The model under review builds one solid part; all positions refer to its coordinate system, in mm. Coordinates: 2 decimals unless noted, no trailing zeros. Order: outer loops, then holes, each group sorted by start corner. A loop starts at its lowest first (then second) coordinate and runs counter-clockwise, first axis right, second up. Notation, with made-up numbers: M 54.5,3 L 74.5,3 A25 cw 74.5,20 Z; hole C 41,10 d7. An arc over 180 degrees is marked long. Answer as CSV lines item,"result". Start each with the question number.
Q1. For P1, Ø10, axis at x = 14.5, y = 2, coming from the +Z side; P2, Ø2, axis at y = 2, z = 1.5, coming from the -X side (3 decimals); P3, Ø3, axis at y = 9.5, z = 2, coming from the +X side; P4, Ø1, axis at y = 9.5, z = 1.5, coming from the +X side, all flat-tipped, find the tip position at first contact; note any pin that passes through.
Q2. Wall thickness on L1, parallel to X at y = 15.5, z = 2.25; L2, parallel to Y at x = 7.5, z = 2.25; L3, parallel to Y at x = -11.5, z = 4.9: over which ranges is each line inside the solid? List them lowest first. Write a range as [from, to].
Q3. Consider section B-B on y = 5. Write out the cut boundary in (x, z), and give its area (3 significant figures).
Q4. Consider section A-A on x = 0. Write out the cut boundary in (y, z).
Q5. Consider section C-C on y = -8.5. Write out the cut boundary in (x, z), and give its area (3 significant figures).
Q6. Consider section D-D on x = -8. Write out the cut boundary in (y, z).
from build123d import *

# Parameters (mm, degrees)
SKETCH1_R           = 20
BOSS_EXTRUDE1_DEPTH = 6


with BuildPart() as part:
    # Sketch1 → Boss-Extrude1 (new body)
    with BuildSketch(Plane.XY):
        Circle(SKETCH1_R)
        with BuildLine():
            Line((-2, -2.236067977), (2, -2.236067977))
            ThreePointArc((2, -2.236067977), (0, 3), (-2, -2.236067977))
        make_face(mode=Mode.SUBTRACT)
        with BuildLine():
            Line((-16.568425726, -3.806214518), (-5.988664565, -0.368641735))
            ThreePointArc((-5.988664565, -0.368641735), (-6, 0), (-5.988664565, 0.368641735))
            Line((-5.988664565, 0.368641735), (-16.568425726, 3.806214518))
            ThreePointArc((-16.568425726, 3.806214518), (-17, 0), (-16.568425726, -3.806214518))
        make_face(mode=Mode.SUBTRACT)
        with BuildLine():
            Line((-1.5, -16.933694222), (-1.5, -5.809475019))
            ThreePointArc((-1.5, -5.809475019), (-1.854101966, -5.706339098), (-2.201198248, -5.581641897))
            Line((-2.201198248, -5.581641897), (-8.739850239, -14.581324281))
            ThreePointArc((-8.739850239, -14.581324281), (-5.253288904, -16.167960777), (-1.5, -16.933694222))
        make_face(mode=Mode.SUBTRACT)
        with BuildLine():
            Line((1.5, -16.933694222), (1.5, -5.809475019))
            ThreePointArc((1.5, -5.809475019), (1.854101966, -5.706339098), (2.201198248, -5.581641897))
            Line((2.201198248, -5.581641897), (8.739850239, -14.581324281))
            ThreePointArc((8.739850239, -14.581324281), (5.253288904, -16.167960777), (1.5, -16.933694222))
        make_face(mode=Mode.SUBTRACT)
        with BuildLine():
            Line((-1.5, 5.809475019), (-1.5, 16.933694222))
            ThreePointArc((-1.5, 16.933694222), (-5.253288904, 16.167960777), (-8.739850239, 14.581324281))
            Line((-8.739850239, 14.581324281), (-2.201198248, 5.581641897))
            ThreePointArc((-2.201198248, 5.581641897), (-1.854101966, 5.706339098), (-1.5, 5.809475019))
        make_face(mode=Mode.SUBTRACT)
        with BuildLine():
            Line((-5.061613582, 3.221811284), (-15.641374743, 6.659384067))
            ThreePointArc((-15.641374743, 6.659384067), (-13.753288904, 9.992349289), (-11.166901222, 12.817968525))
            Line((-11.166901222, 12.817968525), (-4.628249231, 3.818286141))
            ThreePointArc((-4.628249231, 3.818286141), (-4.854101966, 3.526711514), (-5.061613582, 3.221811284))
        make_face(mode=Mode.SUBTRACT)
        with BuildLine():
            Line((-15.641374743, -6.659384067), (-5.061613582, -3.221811284))
            ThreePointArc((-5.061613582, -3.221811284), (-4.854101966, -3.526711514), (-4.628249231, -3.818286141))
            Line((-4.628249231, -3.818286141), (-11.166901222, -12.817968525))
            ThreePointArc((-11.166901222, -12.817968525), (-13.753288904, -9.992349289), (-15.641374743, -6.659384067))
        make_face(mode=Mode.SUBTRACT)
        with BuildLine():
            Line((11.166901222, 12.817968525), (4.628249231, 3.818286141))
            ThreePointArc((4.628249231, 3.818286141), (4.854101966, 3.526711514), (5.061613582, 3.221811284))
            Line((5.061613582, 3.221811284), (15.641374743, 6.659384067))
            ThreePointArc((15.641374743, 6.659384067), (13.753288904, 9.992349289), (11.166901222, 12.817968525))
        make_face(mode=Mode.SUBTRACT)
        with BuildLine():
            Line((8.739850239, 14.581324281), (2.201198248, 5.581641897))
            ThreePointArc((2.201198248, 5.581641897), (1.854101966, 5.706339098), (1.5, 5.809475019))
            Line((1.5, 5.809475019), (1.5, 16.933694222))
            ThreePointArc((1.5, 16.933694222), (5.253288904, 16.167960777), (8.739850239, 14.581324281))
        make_face(mode=Mode.SUBTRACT)
        with BuildLine():
            Line((15.641374743, -6.659384067), (5.061613582, -3.221811284))
            ThreePointArc((5.061613582, -3.221811284), (4.854101966, -3.526711514), (4.628249231, -3.818286141))
            Line((4.628249231, -3.818286141), (11.166901222, -12.817968525))
            ThreePointArc((11.166901222, -12.817968525), (13.753288904, -9.992349289), (15.641374743, -6.659384067))
        make_face(mode=Mode.SUBTRACT)
        with BuildLine():
            Line((16.568425726, -3.806214518), (5.988664565, -0.368641735))
            ThreePointArc((5.988664565, -0.368641735), (6, 0), (5.988664565, 0.368641735))
            Line((5.988664565, 0.368641735), (16.568425726, 3.806214518))
            ThreePointArc((16.568425726, 3.806214518), (17, 0), (16.568425726, -3.806214518))
        make_face(mode=Mode.SUBTRACT)
    extrude(amount=BOSS_EXTRUDE1_DEPTH)


solid = part.part
Evaluation:
1,P1,"stops at z = 6"
1,P2,"stops at x = -19.975"
1,P3,"stops at x = 18.33"
1,P4,"stops at x = 17.86"
2,L1,"x = [-12.64, -6.98], [-1.5, 1.5], [6.98, 12.64]"
2,L2,"y = [-18.54, -15.26], [-12.87, -7.77], [-4.01, -0.86], [0.86, 4.01], [7.77, 12.87], [15.26, 18.54]"
2,L3,"y = [-16.36, -12.52], [-5.31, -2.16], [2.16, 5.31], [12.52, 16.36]"
3,outline,"M -19.36,0 L -10.53,0 L -10.53,6 L -19.36,6 Z; M -5.49,0 L 5.49,0 L 5.49,6 L -5.49,6 Z; M 10.53,0 L 19.36,0 L 19.36,6 L 10.53,6 Z"
3,area,"172 mm²"
4,outline,"M -20,0 L -2.24,0 L -2.24,6 L -20,6 Z; M 3,0 L 20,0 L 20,6 L 3,6 Z"
5,outline,"M -18.1,0 L -14.72,0 L -14.72,6 L -18.1,6 Z; M -8.03,0 L -4.32,0 L -4.32,6 L -8.03,6 Z; M -1.5,0 L 1.5,0 L 1.5,6 L -1.5,6 Z; M 4.32,0 L 8.03,0 L 8.03,6 L 4.32,6 Z; M 14.72,0 L 18.1,0 L 18.1,6 L 14.72,6 Z"
5,area,"103 mm²"
6,outline,"M -18.33,0 L -15,0 L -15,6 L -18.33,6 Z; M -13.56,0 L -8.46,0 L -8.46,6 L -13.56,6 Z; M -4.18,0 L -1.02,0 L -1.02,6 L -4.18,6 Z; M 1.02,0 L 4.18,0 L 4.18,6 L 1.02,6 Z; M 8.46,0 L 13.56,0 L 13.56,6 L 8.46,6 Z; M 15,0 L 18.33,0 L 18.33,6 L 15,6 Z"
